```python
from build123d import *

# Parameters (mm, degrees)
BOSS_EXTRUDE1_DEPTH     = 50
CUT_EXTRUDE6_DEPTH      = 25
CUT_EXTRUDE3_DEPTH      = 39.00000000000001
SKETCH14_R              = 7.5000000000001545
BOSS_EXTRUDE7_DEPTH     = 7
SKETCH15_R              = 2.800000000000002
CUT_EXTRUDE4_DEPTH      = 27.999999999999996
SKETCH16_R              = 5.249999999999997
CUT_EXTRUDE5_DEPTH      = 1.5
CUT_EXTRUDE7_DEPTH      = 54.52569476429079
SKETCH19_R              = 2.1499999999999995
CUT_EXTRUDE9_DEPTH      = 50
ENL_V_MAT_EXTRU_1_DEPTH = 7.5
ENL_V_MAT_EXTRU_3_DEPTH = 10
BOSS_EXTRU_1_DEPTH      = 26.00000000000001
ENL_V_MAT_EXTRU_5_DEPTH = 3.5
BOSS_EXTRU_3_DEPTH      = 1
BOSS_EXTRU_4_START      = -5.8
BOSS_EXTRU_4_DEPTH      = 5.8
BOSS_EXTRU_5_DEPTH      = 0.1
BOSS_EXTRU_6_DEPTH      = 0.1
ESQUISSE13_W            = 6.549999999999918
ESQUISSE13_H            = 9.750000000000139
BOSS_EXTRU_7_DEPTH      = 3.6
ESQUISSE14_W            = 6.549999999999992
ESQUISSE14_H            = 9.750000000000139
BOSS_EXTRU_8_DEPTH      = 3.6
BOSS_EXTRU_11_DEPTH     = 25
BOSS_EXTRU_12_DEPTH     = 25
ENL_V_MAT_EXTRU_6_DEPTH = 28.00000000000001
CONG_1_R                = 3


with BuildPart() as part:
    # Sketch1 → Boss-Extrude1 (new body)
    with BuildSketch(Plane(origin=(0, 0, 0), x_dir=(1, 0, 0), z_dir=(0, 1, 0))):
        Polygon((-13.000000000000004, 14), (12.999999999999996, 14), (13.000000000000002, -14), (-12.999999999999998, -14), align=None)
    extrude(amount=BOSS_EXTRUDE1_DEPTH)

    # Sketch3 → Cut-Extrude6 (cut)
    with BuildSketch(Plane(origin=(0, 0, 0), x_dir=(1, 0, 0), z_dir=(0, 1, 0))):
        Polygon((9.998973293230602, 2.6500000000000012), (9.9989732932306, 9.850000000000001), (2.9002540058261537, 9.850000000000001), (2.881158297661572, 5.82281627717582), (-2.9187777922427904, 5.850044075927868), (-2.8999999999999972, 9.850000000000001), (-9.999999999999996, 9.85), (-9.999999999999995, 2.6499999999999995), (-8.99999999999974, 2.6499999999999995), (-6.00000000000001, -3.2500000000000027), (-9.999999999999998, -3.2500000000000027), (-9.999999999999993, -4.349999999999079), (-9.99999999999999, -15.089504782389637), (10.190019105374848, -15.102048820223754), (10.123266065424222, -8.899331206040385), (10.06892160658641, -3.849623622447693), (10.062468515842252, -3.2500000000000027), (6.072889948170096, -3.2500000000000027), (8.998973293230604, 2.6500000000000017), align=None)
    extrude(amount=CUT_EXTRUDE6_DEPTH, mode=Mode.SUBTRACT)

    # Sketch7 → Cut-Extrude3 (cut)
    with BuildSketch(Plane(origin=(13, 0, -2.42e-15), x_dir=(-1.3e-16, 0, -1), z_dir=(1, 0, -1.3e-16))):
        with BuildLine():
            Line((4.499999999999999, 50), (-14.000000000000002, 50))
            Line((-14.000000000000002, 50), (-14.000000000000002, 24.000000000000004))
            Line((-14.000000000000002, 24.000000000000004), (-0.8033008588991847, 37.19669914110098))
            ThreePointArc((-0.8033008588991847, 37.19669914110098), (11.429096493834622, 39.629874257261775), (4.499999999999999, 50))
        make_face()
    extrude(amount=-CUT_EXTRUDE3_DEPTH, mode=Mode.SUBTRACT)

    # Sketch14 → Boss-Extrude7 (add)
    with BuildSketch(Plane(origin=(13, 0, -2.42e-15), x_dir=(-1.3e-16, 0, -1), z_dir=(1, 0, -1.3e-16))):
        with Locations((4.499999999999999, 42.500000000000114)):
            Circle(SKETCH14_R)
    boss_extrude7 = extrude(amount=-BOSS_EXTRUDE7_DEPTH)

    # Symétrie1: Boss-Extrude7 across plane
    add(boss_extrude7.mirror(Plane(origin=(0, 0, 0), x_dir=(0, 0, 1), z_dir=(1, 0, 0))))

    # Sketch15 → Cut-Extrude4 (cut)
    with BuildSketch(Plane(origin=(13, 0, -2.42e-15), x_dir=(-1.3e-16, 0, -1), z_dir=(1, 0, -1.3e-16))):
        with Locations((4.499999999999999, 42.50000000000027)):
            Circle(SKETCH15_R)
    extrude(amount=-CUT_EXTRUDE4_DEPTH, mode=Mode.SUBTRACT)

    # Sketch16 → Cut-Extrude5 (cut)
    with BuildSketch(Plane(origin=(13, 0, -2.42e-15), x_dir=(-1.3e-16, 0, -1), z_dir=(1, 0, -1.3e-16))):
        with Locations((4.499999999999999, 42.50000000000027)):
            Circle(SKETCH16_R)
    cut_extrude5 = extrude(amount=-CUT_EXTRUDE5_DEPTH, mode=Mode.SUBTRACT)

    # Mirror3: Cut-Extrude5 across plane
    add(cut_extrude5.mirror(Plane(origin=(0, 0, 0), x_dir=(0, 0, 1), z_dir=(1, 0, 0))), mode=Mode.SUBTRACT)

    # Sketch17 → Cut-Extrude7 (cut, through all)
    with BuildSketch(Plane.XZ):
        Polygon((-9.29999999999996, 3.250000000000054), (-13.000000000000009, 3.2500000000000546), (-12.999999999999998, 14), (13.000000000000002, 14), (12.99999999999999, 3.2500000000000546), (9.300000000000033, 3.2499999999999205), (9.300000000000033, 9.79999999999992), (-9.29999999999996, 9.80000000000005), align=None)
    extrude(amount=-CUT_EXTRUDE7_DEPTH, mode=Mode.SUBTRACT)

    # Sketch19 → Cut-Extrude9 (cut)
    with BuildSketch(Plane(origin=(0, 0, -14), x_dir=(-1, 0, 0), z_dir=(0, 0, -1))):
        with Locations((0, 15)):
            Circle(SKETCH19_R)
    extrude(amount=-CUT_EXTRUDE9_DEPTH, mode=Mode.SUBTRACT)

    # Esquisse1 → Enlèv. mat.-Extru.1 (cut)
    with BuildSketch(Plane(origin=(0, 50, 0), x_dir=(1, 0, 0), z_dir=(0, 1, 0))):
        Polygon((5.999999999999998, 4.500000000000001), (-6.000000000000002, 4.499999999999999), (-6, 14), (5.999999999999998, 14), align=None)
    extrude(amount=-ENL_V_MAT_EXTRU_1_DEPTH, mode=Mode.SUBTRACT)

    # Esquisse3 → Enlèv. mat.-Extru.3 (cut)
    with BuildSketch(Plane(origin=(0, 0, -14), x_dir=(-1, 0, 0), z_dir=(0, 0, -1))):
        Polygon((6, 42.5), (-6, 42.5), (-5.999999999999999, 35), (6.000000000000001, 35), align=None)
    extrude(amount=-ENL_V_MAT_EXTRU_3_DEPTH, mode=Mode.SUBTRACT)

    # Esquisse6 → Boss.-Extru.1 (add)
    with BuildSketch(Plane(origin=(13, 0, -2.42e-15), x_dir=(-1.9e-16, 0, -1), z_dir=(1, 0, -1.9e-16))):
        with BuildLine():
            Line((-3.2500000000000573, 34.75000000000014), (-3.2500000000000573, 42.50000000000006))
            Line((-3.2500000000000573, 42.50000000000006), (-3.0000000000000226, 42.50000000000006))
            ThreePointArc((-3.0000000000000226, 42.50000000000006), (-2.4290964938347503, 39.629874257261875), (-0.8033008588992404, 37.19669914110092))
            Line((-0.8033008588992404, 37.19669914110092), (-3.2500000000000573, 34.75000000000014))
        make_face()
    extrude(amount=-BOSS_EXTRU_1_DEPTH)

    # Esquisse7 → Enlèv. mat.-Extru.5 (cut)
    with BuildSketch(Plane(origin=(0, 42.50000000000006, 0), x_dir=(1, 0, 0), z_dir=(0, 1, 0))):
        Polygon((5.999999999999993, -3.0000000000000213), (5.999999999999993, -7.096354864410982), (-6.000000000000002, -3.7800697907913037), (-6.000000000000002, 8.456914552722129), align=None)
    extrude(amount=-ENL_V_MAT_EXTRU_5_DEPTH, mode=Mode.SUBTRACT)

    # Esquisse9 → Boss.-Extru.3 (add)
    with BuildSketch(Plane(origin=(0, 25, 0), x_dir=(-1, 0, 0), z_dir=(0, -1, 0))):
        Polygon((2.899999999999959, -9.80000000000005), (-2.9000000000000408, -9.80000000000005), (-2.9000000000000408, -6.8000000000000504), (2.899999999999959, -6.80000000000005), align=None)
    extrude(amount=BOSS_EXTRU_3_DEPTH)

    # Esquisse10 → Boss.-Extru.4 (add)
    with BuildSketch(Plane.ZY.offset(2.899999999999959).offset(BOSS_EXTRU_4_START)):
        Polygon((9.80000000000005, 24), (9.80000000000005, 22), (6.80000000000005, 24), align=None)
    extrude(amount=BOSS_EXTRU_4_DEPTH)

    # Esquisse11 → Boss.-Extru.5 (add)
    with BuildSketch(Plane.ZY.offset(9.29999999999996)):
        Polygon((3.2500000000000586, 34.75000000000014), (9.80000000000005, 28.20000000000007), (9.80000000000005, 25), (3.2500000000000586, 25), align=None)
    extrude(amount=BOSS_EXTRU_5_DEPTH)

    # Esquisse12 → Boss.-Extru.6 (add)
    with BuildSketch(Plane(origin=(9.300000000000033, 0, 0), x_dir=(0, 0, -1), z_dir=(1, 0, 0))):
        Polygon((-9.79999999999992, 25), (-9.799999999999923, 28.20000000000013), (-3.250000000000055, 34.75000000000014), (-3.2499999999999205, 25), align=None)
    extrude(amount=BOSS_EXTRU_6_DEPTH)

    # Esquisse13 → Boss.-Extru.7 (add)
    with BuildSketch(Plane(origin=(9.400000000000032, 0, 0), x_dir=(0, 0, -1), z_dir=(1, 0, 0))):
        with Locations((-6.524999999999961, 29.87500000000007)):
            Rectangle(ESQUISSE13_W, ESQUISSE13_H)
    extrude(amount=BOSS_EXTRU_7_DEPTH)

    # Esquisse14 → Boss.-Extru.8 (add)
    with BuildSketch(Plane.ZY.offset(9.39999999999996)):
        with Locations((6.5250000000000545, 29.87500000000007)):
            Rectangle(ESQUISSE14_W, ESQUISSE14_H)
    extrude(amount=BOSS_EXTRU_8_DEPTH)

    # Esquisse18 → Boss.-Extru.11 (add)
    with BuildSketch(Plane.XZ):
        Polygon((-13.000000000000009, 3.2500000000000524), (-33.35159698893457, -32), (33.35159698893456, -32), (12.99999999999999, 3.2500000000000546), (12.999999999999996, -14), (-13.000000000000004, -14), align=None)
    extrude(amount=-BOSS_EXTRU_11_DEPTH)

    # Esquisse19 → Boss.-Extru.12 (add)
    with BuildSketch(Plane(origin=(0, 25, 0), x_dir=(1, 0, 0), z_dir=(0, 1, 0))):
        Polygon((33.35159698893456, 32), (22.959292143521182, 14.000000000000002), (-22.95929214352119, 14), (-33.35159698893457, 32), align=None)
    extrude(amount=BOSS_EXTRU_12_DEPTH)

    # Esquisse20 → Enlèv. mat.-Extru.6 (cut)
    with BuildSketch(Plane(origin=(13, 0, -2.42e-15), x_dir=(-1.9e-16, 0, -1), z_dir=(1, 0, -1.9e-16))):
        Polygon((14, 25), (14, 50), (19, 50), align=None)
    enl_v_mat_extru_6 = extrude(amount=ENL_V_MAT_EXTRU_6_DEPTH, mode=Mode.SUBTRACT)

    # Symétrie3: Enlèv. mat.-Extru.6 across plane
    add(enl_v_mat_extru_6.mirror(Plane(origin=(0, 0, 0), x_dir=(0, 0, 1), z_dir=(1, 0, 0))), mode=Mode.SUBTRACT)

    # Congé1
    cong_1_edges = [part.edges().sort_by_distance(p)[0] for p in [
        (33.35159698893456, 25, -32),
        (-33.35159698893457, 25, -32),
        (-7.11e-15, 50, -32),
    ]]
    fillet(cong_1_edges, radius=CONG_1_R)


solid = part.part
```
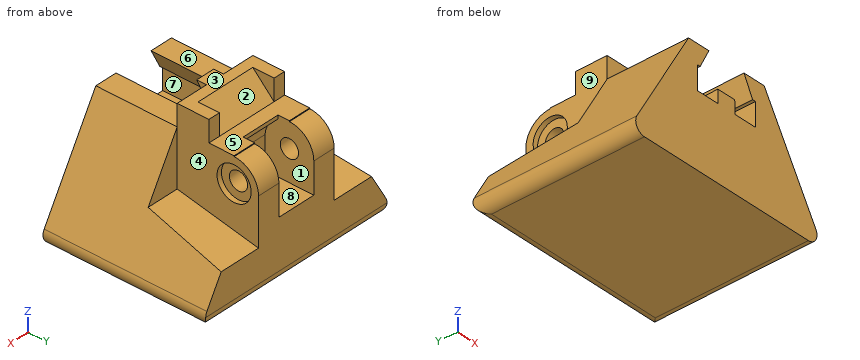
Could you check a few things on this model? Use its own coordinates, in mm. Face numbers are marked on the shaded views. A direction names the side the tool comes from. Round coordinates to 2 decimals unless told otherwise and drop trailing zeros. Loops run counter-clockwise (first coordinate to the right, second up) from the corner with the lowest first, then second, coordinate; pieces in that order, holes last. Notation, with made-up numbers: M 39,22 L 52,22 A10 cw 52,26 Z; hole C 11.5,76 d2. An arc over 180 degrees is marked long. Answer as CSV lines item,"result".
1) Which directions (+Z, -Z, +X, -X, +Y, -Y) give clear straight access to the entire face, cutting with the end or side of a thin tool? Please do the marked faces 5, 6, 7, 8 and 9.
From the geometry:
face 5,"+Z, +X, -X, +Y"
face 6,"+Z, +X, -X, -Y"
face 7,"-Y"
face 8,"+Y"
face 9,"+Z, -X, +Y"
2) Imagine slicing it at B-B on z = 4. List the corners of the cut face in (x, y) for me, and give its area (3 significant figures).
From the geometry:
outline,"M -13,25 L 13,25 L 13,34.75 L 9.4,34.75 L 9.4,34 L -9.4,34 L -9.4,34.75 L -13,34.75 Z"
area,"239 mm^2"
3) Imagine slicing it at A-A on y = 19. List the corners of the cut face in (x, z) for me, and give its area (3 significant figures).
From the geometry:
outline,"M -30.75,-27.5 A3 ccw -28.16,-32 L 28.16,-32 A3 ccw 30.75,-27.5 L 13,3.25 L 6.07,3.25 L 9,-2.65 L 10,-2.65 L 10,-9.85 L 2.9,-9.85 L 2.88,-5.82 L -2.92,-5.85 L -2.9,-9.85 L -10,-9.85 L -10,-2.65 L -9,-2.65 L -6,3.25 L -13,3.25 Z"
area,"1,410 mm^2"
4) We'd pull the mould along X, two halves only. Please class the marked faces 1, 2, 3 and 4: released by +X, released by -X, zero draft, split by the parting line, or undercut.
From the geometry:
face 1,"undercut"
face 2,"undercut"
face 3,"zero draft"
face 4,"released by +X"
5) If I drill on probe 1 along Y at (x, z) = (12.6, -4.5); probe 2 along Z at (x, y) = (2, 21.5); probe 3 along Y at (x, z) = (0, -11), over which ranges is the centre line in solid material (lowest first)?
From the geometry:
probe 1,"0 to 37.25, 47.75 to 50"
probe 2,"-32 to -5.83"
probe 3,"0 to 12.85, 17.15 to 35"
6) For pin 1 Ø11 at (x, z) = (19, -7) entering from +Y; pin 2 Ø1 at (y, z) = (13.5, 4) entering from -X; pin 3 Ø1 at (y, z) = (19.5, -16) entering from +X; pin 4 Ø13.5 at (y, z) = (42.5, -4.5) entering from +X, each with a flat end and sliding along its axis, tell me the tip position at first contact or that it passes through.
From the geometry:
pin 1,"y = 25"
pin 2,"through"
pin 3,"x = 24.4"
pin 4,"x = 13"
7) Imagine slicing it at D-D on x = 19. List the corners of the cut face in (y, z) for me, and give its area (3 significant figures).
From the geometry:
outline,"M 0,-32 L 47,-32 A3 ccw 50,-29 L 50,-19 L 25,-14 L 25,-7.14 L 0,-7.14 Z"
area,"1,010 mm^2"
